Can you work these out from the drawing? Everything is in mm from the part's minimum corner. A direction names the side the tool comes from. Coordinates: 2 decimals unless noted, no trailing zeros. Loops run counter-clockwise (first coordinate to the right, second up) from the corner with the lowest first, then second, coordinate; pieces in that order, holes last. Notation, with made-up numbers: (78.5, -29.75) - (104.5, -29.75) arc R8 ccw to (104.5, -19.75) - close; hole circle Ø5 at (-29.5, 60.5). An arc over 180 degrees is marked (long way). Put each result on its own line as item: value. Start each with the question number.
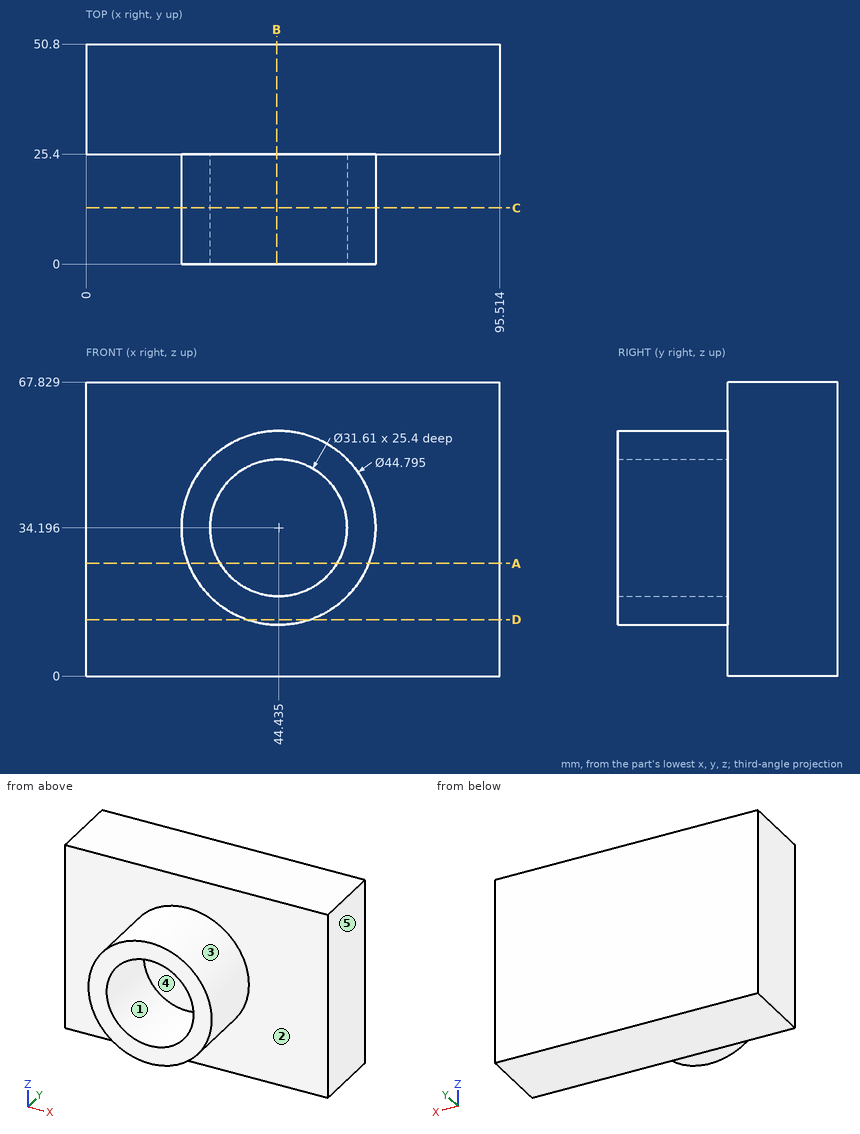
(1) I want a section at A-A on z = 26. List the corners of the cut face in (x, y) for me, and give its area (3 significant figures).
(2) I need wall thicknesses on L1, parallel to Y at x = 20.5, z = 61; L2, parallel to X at y = 19.5, z = 21 (1 decimal); L3, parallel to Z at x = 41, y = 5. Which ranges of each line are inside material? Lowest first, please. Write a range as [from, to].
(3) I want a section at B-B on x = 44. List the corners of the cut face in (y, z) for me (1 decimal), and give its area (3 significant figures).
(4) Which directions (+Z, -Z, +X, -X, +Y, -Y) give clear straight access to the entire face, cutting with the end or side of a thin tool? Please do the marked faces 4 and 5.
(5) If we mould it in two halves opening along Z, with no side actions, what happens to the marked faces 1, 2 and 3? For each: pulls with the +Z half, pulls with the -Z half, needs draft (parallel to the pull), parting line crosses it, or undercut.
(6) For pin 1 Ø10 at (x, z) = (69.5, 10.5) entering from -Y; pin 2 Ø1.5 at (y, z) = (8.5, 33) entering from +X; pin 3 Ø4 at (x, y) = (61, 20) entering from +Z, each with a flat end and sliding along its axis, tell me the tip position at first contact or that it passes through.
(7) I want a section at D-D on z = 13. List the corners of the cut face in (x, y) for me, and give its area (3 significant figures).
(8) I want a section at C-C on y = 13. List the corners of the cut face in (x, z) for me (1 decimal), and give its area (3 significant figures).
Answer sheet:
1. outline: (0, 25.4) - (23.59, 25.4) - (23.59, 0) - (30.92, 0) - (30.92, 25.4) - (57.95, 25.4) - (57.95, 0) - (65.28, 0) - (65.28, 25.4) - (95.51, 25.4) - (95.51, 50.8) - (0, 50.8) - close
1. area: 2,800 mm^2
2. L1: y = [25.4, 50.8]
2. L2: x = [26.3, 35.7], [53.1, 62.5]
2. L3: z = [12.06, 18.77], [49.62, 56.33]
3. outline: (0, 11.8) - (25.4, 11.8) - (25.4, 0) - (50.8, 0) - (50.8, 67.8) - (25.4, 67.8) - (25.4, 56.6) - (0, 56.6) - (0, 50) - (25.4, 50) - (25.4, 18.4) - (0, 18.4) - close
3. area: 2,060 mm^2
4. face 4: -Y
4. face 5: +Z, -Z, +X, +Y, -Y
5. face 1: undercut
5. face 2: needs draft
5. face 3: parting line crosses it
6. pin 1: stops at y = 25.4
6. pin 2: stops at x = 66.83
6. pin 3: stops at z = 51.21
7. outline: (0, 25.4) - (37.2, 25.4) - (37.2, 0) - (51.67, 0) - (51.67, 25.4) - (95.51, 25.4) - (95.51, 50.8) - (0, 50.8) - close
7. area: 2,790 mm^2
8. outline: circle Ø44.8 at (44.4, 34.2); hole circle Ø31.6 at (44.4, 34.2)
8. area: 791 mm^2
